Work out the finished part from the listing and answer in its coordinate system (mm). Face numbers are marked on the shaded views. A direction names the side the tool comes from. Coordinates: 2 decimals unless noted, no trailing zeros. Order: outer loops, then holes, each group sorted by start corner. A loop starts at its lowest first (then second) coordinate and runs counter-clockwise, first axis right, second up. Notation, with made-up numbers: M 6,51.25 L 63,51.25 A23 ccw 63,59.25 Z; hole C -6.5,36 d1. An arc over 180 degrees is marked long. Use a Markdown table: item, result.
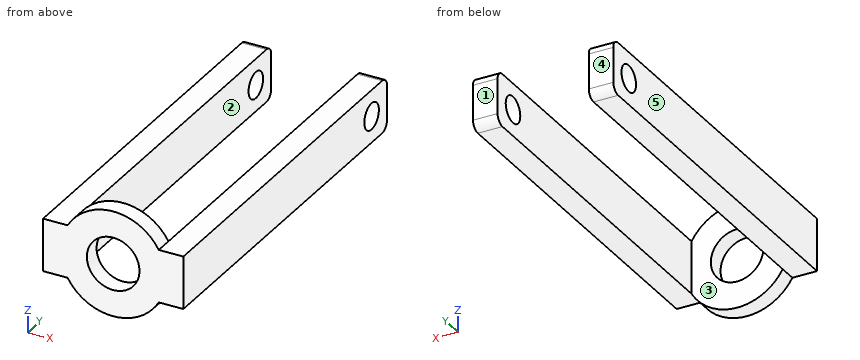
from build123d import *

# Parameters (mm, degrees)
BOSS_EXTRUDE1_DEPTH = 100
SKETCH2_W           = 140.192378865
SKETCH2_H           = 300
BOSS_EXTRUDE2_DEPTH = 2000
SKETCH3_R           = 150
CUT_EXTRUDE1_DEPTH  = 100
FILLET1_R           = 50
CUT_EXTRUDE2_START  = -800
SKETCH4_R           = 75
CUT_EXTRUDE2_DEPTH  = 800


with BuildPart() as part:
    # Sketch1 → Boss-Extrude1 (new body)
    with BuildSketch(Plane(origin=(0, 0, 0), x_dir=(1, 0, 0), z_dir=(0, 1, 0))):
        with BuildLine():
            ThreePointArc((259.807621135, 150), (0, 300), (-259.807621135, 150))
            Line((-259.807621135, 150), (259.807621135, 150))
        make_face()
        with BuildLine():
            Line((259.807621135, 150), (-259.807621135, 150))
            ThreePointArc((-259.807621135, 150), (-300, 0), (-259.807621135, -150))
            Line((-259.807621135, -150), (259.807621135, -150))
            ThreePointArc((259.807621135, -150), (289.777747887, -77.645713531), (300, 0))
            ThreePointArc((300, 0), (289.777747887, 77.645713531), (259.807621135, 150))
        make_face()
        with BuildLine():
            Line((259.807621135, -150), (-259.807621135, -150))
            ThreePointArc((-259.807621135, -150), (0, -300), (259.807621135, -150))
        make_face()
        with BuildLine():
            Line((-259.807621135, 150), (-400, 150))
            Line((-400, 150), (-400, -150))
            Line((-400, -150), (-259.807621135, -150))
            ThreePointArc((-259.807621135, -150), (-300, 0), (-259.807621135, 150))
        make_face()
        with BuildLine():
            Line((400, 150), (259.807621135, 150))
            ThreePointArc((259.807621135, 150), (289.777747887, 77.645713531), (300, 0))
            ThreePointArc((300, 0), (289.777747887, -77.645713531), (259.807621135, -150))
            Line((259.807621135, -150), (400, -150))
            Line((400, -150), (400, 150))
        make_face()
    extrude(amount=BOSS_EXTRUDE1_DEPTH)

    # Sketch2 → Boss-Extrude2 (add)
    with BuildSketch(Plane(origin=(0, 100, 0), x_dir=(1, 0, 0), z_dir=(0, 1, 0))):
        with Locations((-329.903810568, 0)):
            Rectangle(SKETCH2_W, SKETCH2_H)
        with Locations((329.903810568, 0)):
            Rectangle(SKETCH2_W, SKETCH2_H)
    extrude(amount=BOSS_EXTRUDE2_DEPTH)

    # Sketch3 → Cut-Extrude1 (cut)
    with BuildSketch(Plane(origin=(0, 100, 0), x_dir=(1, 0, 0), z_dir=(0, 1, 0))):
        with Locations(Location((0, 0, 0), (0, 0, 270))):
            Circle(SKETCH3_R)
    extrude(amount=-CUT_EXTRUDE1_DEPTH, mode=Mode.SUBTRACT)

    # Fillet1
    fillet1_edges = [part.edges().sort_by_distance(p)[0] for p in [
        (-329.903810568, 2100, -150),
        (-329.903810568, 2100, 150),
        (329.903810568, 2100, -150),
        (329.903810568, 2100, 150),
    ]]
    fillet(fillet1_edges, radius=FILLET1_R)

    # Sketch4 → Cut-Extrude2 (cut)
    with BuildSketch(Plane.ZY.offset(400).offset(CUT_EXTRUDE2_START)):
        with Locations((0, 1941.16)):
            Circle(SKETCH4_R)
    extrude(amount=CUT_EXTRUDE2_DEPTH, mode=Mode.SUBTRACT)


solid = part.part
1. Section C-C on y = 1298 is taken. Determine the outline of the cut face in (x, z), then the cut area to 3 significant figures.
Answers below:
| item | result |
|---|---|
| outline | M -400,-150 L -259.81,-150 L -259.81,150 L -400,150 Z; M 259.81,-150 L 400,-150 L 400,150 L 259.81,150 Z |
| area | 84,100 mm² |
2. Section D-D on y = 1941.16 is taken. Determine the outline of the cut face in (x, z), then the cut area to 3 significant figures.
Answers below:
| item | result |
|---|---|
| outline | M -400,-150 L -259.81,-150 L -259.81,-75 L -400,-75 Z; M -400,75 L -259.81,75 L -259.81,150 L -400,150 Z; M 259.81,-150 L 400,-150 L 400,-75 L 259.81,-75 Z; M 259.81,75 L 400,75 L 400,150 L 259.81,150 Z |
| area | 42,100 mm² |
3. Find the intervals of material crossed by probe 1 along X at (y, z) = (435, -22.5); probe 2 along Z at (x, y) = (-315, 1941); probe 3 along Y at (x, z) = (-320, 0), in increasing order.
Answers below:
| item | result |
|---|---|
| probe 1 | -400 to -259.81, 259.81 to 400 |
| probe 2 | -150 to -75, 75 to 150 |
| probe 3 | 0 to 1866.16, 2016.16 to 2100 |
4. Section A-A on x = 0 is taken. Determine the outline of the cut face in (y, z), then the cut area to 3 significant figures.
Answers below:
| item | result |
|---|---|
| outline | M 0,-300 L 100,-300 L 100,-150 L 0,-150 Z; M 0,150 L 100,150 L 100,300 L 0,300 Z |
| area | 30,000 mm² |
5. For a pull along X with two mould halves and no side action, classify the marked faces 3, 4 and 5 as +X half, -X half, draft (parallel to the pull), parting line (faces both ways), or undercut.
Answers below:
| item | result |
|---|---|
| face 3 | undercut |
| face 4 | draft |
| face 5 | -X half |
6. A flat-ended cylindrical pin translates along its axis: P1, Ø12, axis at x = -12, z = -167, coming from the +Y side. Find the tip coordinate at first contact, or state that the pin passes through.
Answers below:
| item | result |
|---|---|
| P1 | y = 100 |
7. For the marked faces 1 and 2, determine the directions among +Z, -Z, +X, -X, +Y, -Y from which every point of the face is accessible in a straight line to the end or side of a thin tool.
Answers below:
| item | result |
|---|---|
| face 1 | +Z, -Z, +X, -X, +Y |
| face 2 | +Z, -Z, +Y |
8. Section B-B on z = 0 is taken. Determine the outline of the cut face in (x, y).
Answers below:
| item | result |
|---|---|
| outline | M -400,0 L -150,0 L -150,100 L -259.81,100 L -259.81,1866.16 L -400,1866.16 Z; M -400,2016.16 L -259.81,2016.16 L -259.81,2100 L -400,2100 Z; M 150,0 L 400,0 L 400,1866.16 L 259.81,1866.16 L 259.81,100 L 150,100 Z; M 259.81,2016.16 L 400,2016.16 L 400,2100 L 259.81,2100 Z |
